```python
from build123d import *

# Parameters (mm, degrees)
SKETCH1_W_MOCK_PCB_W             = 50.8
SKETCH1_W_MOCK_PCB_H             = 304.8
BOSS_EXTRUDE1_DEPTH              = 6.35
F_3_8_16_TAPPED_HOLE1_AT_2_COUNT = 2
F_3_8_16_TAPPED_HOLE1_AT_2_PITCH = 254
SKETCH3_R                        = 7.9375
CUT_EXTRUDE1_DEPTH               = 9.398


with BuildPart() as part:
    # Sketch1 w/mock PCB → Boss-Extrude1 (new body, symmetric)
    with BuildSketch(Plane.XY):
        Rectangle(SKETCH1_W_MOCK_PCB_W, SKETCH1_W_MOCK_PCB_H)
    extrude(amount=BOSS_EXTRUDE1_DEPTH, both=True)

    # Sketch1 → 3/8-16 Tapped Hole1 (revolve, cut)
    with BuildSketch(Plane(origin=(0, -127, 6.35), x_dir=(0, -1, 0), z_dir=(1, 0, 0))):
        Polygon((0, 0), (0, 12.7), (4.7625, 12.7), (4.03225, 11.96975), (4.03225, 0.73025), (4.7625, 0), align=None)
    f_3_8_16_tapped_hole1 = revolve(axis=Axis((0, -127, 12.7), (0, 0, -1)), mode=Mode.SUBTRACT)

    # 3/8-16 Tapped Hole1 at 2: 3/8-16 Tapped Hole1 ×2
    with Locations(*[(0, i * F_3_8_16_TAPPED_HOLE1_AT_2_PITCH, 0) for i in range(1, F_3_8_16_TAPPED_HOLE1_AT_2_COUNT)]):
        add(f_3_8_16_tapped_hole1, mode=Mode.SUBTRACT)

    # Sketch3 → Cut-Extrude1 (cut)
    with BuildSketch(Plane.XY.offset(6.35)):
        Circle(SKETCH3_R)
    extrude(amount=-CUT_EXTRUDE1_DEPTH, mode=Mode.SUBTRACT)


solid = part.part
```
Part model, mm, in its own coordinate system. A direction names the side the tool comes from. Round coordinates to 2 decimals unless told otherwise and drop trailing zeros. Order: outer loops, then holes, each group sorted by start corner. A loop starts at its lowest first (then second) coordinate and runs counter-clockwise, first axis right, second up. Notation, with made-up numbers: M -5.75,34 L 19.25,34 A18 cw 19.25,42 Z; hole C 10,22.25 d6. An arc over 180 degrees is marked long. Put each result on its own line as item: value. Start each with the question number.
1. Tool access for faces 4 (the face through (0, 0, -3.048)), 5 (the face through (-0.18, 131.03, 0.08)): list every direction of +Z, -Z, +X, -X, +Y, -Y with a clear straight run to the whole face (end or side of a thin tool).
2. Drop a flat-ended pin along its axis: pin 1 (6.5 mm diameter, centred on x = 0, y = 127, fed in from +Z). Give the stop position or say it passes through.
3. Slice it at D-D on y = 0. List the corners of the cut face in (x, z).
4. Slice it at B-B on x = 0. List the corners of the cut face in (y, z), then the cut area to 3 significant figures.
5. Drill centre lines: probe 1 along Y at (x, z) = (0, -0.5); probe 2 along X at (y, z) = (127, 2.75); probe 3 along X at (y, z) = (4, 4). Where is each one in solid material? Low to high. Write a range as [from, to].
6. Slice it at A-A on y = -127. List the corners of the cut face in (x, z), then the cut area to 3 significant figures.
7. Two-plate mould, pull along X, no slides. Class faces 1 (the face through (-25.4, -2, 0)), 2 (the face through (-0.18, -122.97, 0.08)), 3 (the face through (0, -152.4, 0)): +X half, -X half, draft (parallel to the pull), parting line (faces both ways), or undercut.
8. Slice it at C-C on z = -0.25. List the corners of the cut face in (x, y) (1 decimal).
Findings:
1. face 4: +Z
1. face 5: +Z, -Z
2. pin 1: through
3. outline: M -25.4,-6.35 L 25.4,-6.35 L 25.4,6.35 L 7.94,6.35 L 7.94,-3.05 L -7.94,-3.05 L -7.94,6.35 L -25.4,6.35 Z
4. outline: M -152.4,-6.35 L -131.76,-6.35 L -131.03,-5.62 L -131.03,5.62 L -131.76,6.35 L -152.4,6.35 Z; M -122.97,-5.62 L -122.24,-6.35 L 122.24,-6.35 L 122.97,-5.62 L 122.97,5.62 L 122.24,6.35 L 7.94,6.35 L 7.94,-3.05 L -7.94,-3.05 L -7.94,6.35 L -122.24,6.35 L -122.97,5.62 Z; M 131.03,-5.62 L 131.76,-6.35 L 152.4,-6.35 L 152.4,6.35 L 131.76,6.35 L 131.03,5.62 Z
4. area: 3,510 mm2
5. probe 1: [-152.4, -131.03], [-122.97, -7.94], [7.94, 122.97], [131.03, 152.4]
5. probe 2: [-25.4, -4.03], [4.03, 25.4]
5. probe 3: [-25.4, -6.86], [6.86, 25.4]
6. outline: M -25.4,-6.35 L -4.76,-6.35 L -4.03,-5.62 L -4.03,5.62 L -4.76,6.35 L -25.4,6.35 Z; M 4.03,-5.62 L 4.76,-6.35 L 25.4,-6.35 L 25.4,6.35 L 4.76,6.35 L 4.03,5.62 Z
6. area: 542 mm2
7. face 1: -X half
7. face 2: undercut
7. face 3: draft
8. outline: M -25.4,-152.4 L 25.4,-152.4 L 25.4,152.4 L -25.4,152.4 Z; hole C 0,0 d15.9; hole C 0,-127 d8.1; hole C 0,127 d8.1
